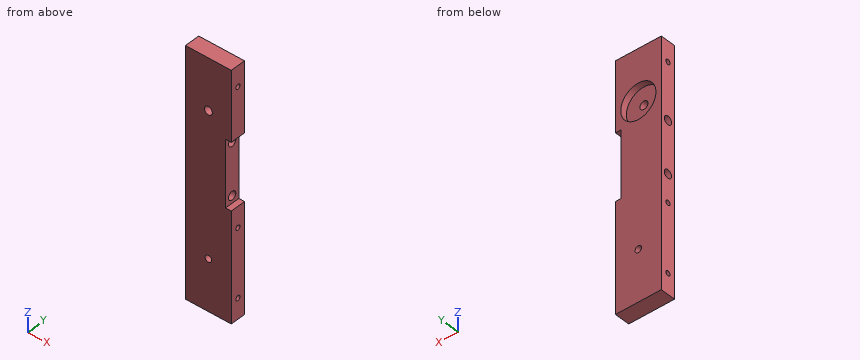
```python
from build123d import *

# Parameters (mm, degrees)
SKETCH2_W             = 28.575
SKETCH2_H             = 152.4
BOSS_EXTRUDE1_DEPTH   = 9.525
F_3_0MM_DOWEL_HOLE1_D = 3
LPATTERN1_COUNT       = 4
LPATTERN1_PITCH       = 42.333333333
SKETCH12_R            = 2.05
CUT_EXTRUDE1_DEPTH    = 156.348048749
SKETCH12_4_R          = 10.975
CUT_EXTRUDE2_DEPTH    = 4
SKETCH15_R            = 2.5
CUT_EXTRUDE3_DEPTH    = 156.154169296
SKETCH13_R            = 2.6
CUT_EXTRUDE4_DEPTH    = 156.348048749
SKETCH17_W            = 41.28
SKETCH17_H            = 9.525
CUT_EXTRUDE5_DEPTH    = 3.575


with BuildPart() as part:
    # Sketch2 → Boss-Extrude1 (new body)
    with BuildSketch(Plane(origin=(0, 0, 0), x_dir=(1, 0, 0), z_dir=(0, 1, 0))):
        with Locations((14.2875, 76.2)):
            Rectangle(SKETCH2_W, SKETCH2_H)
    extrude(amount=BOSS_EXTRUDE1_DEPTH)

    # Ø3.0mm Dowel Hole1 (through all)
    with Locations(Plane.ZY):
        with Locations((-139.7, 4.7625)):
            f_3_0mm_dowel_hole1 = Hole(F_3_0MM_DOWEL_HOLE1_D / 2)

    # LPattern1: Ø3.0mm Dowel Hole1 ×4, 1 skipped
    with Locations(*[(0, 0, i * LPATTERN1_PITCH) for i in range(1, LPATTERN1_COUNT) if i not in (2,)]):
        add(f_3_0mm_dowel_hole1, mode=Mode.SUBTRACT)

    # Sketch12 → Cut-Extrude1 (cut, through all)
    with BuildSketch(Plane(origin=(0, 9.525, 0), x_dir=(1, 0, 0), z_dir=(0, 1, 0))):
        with Locations(Location((14.2875, 120.65, 0), (0, 0, 270))):
            Circle(SKETCH12_R)
    extrude(amount=-CUT_EXTRUDE1_DEPTH, mode=Mode.SUBTRACT)

    # Sketch12<4> → Cut-Extrude2 (cut)
    with BuildSketch(Plane(origin=(0, 9.525, 0), x_dir=(1, 0, 0), z_dir=(0, 1, 0))):
        with Locations(Location((14.2875, 31.75, 0), (0, 0, 270))):
            Circle(SKETCH12_4_R)
    extrude(amount=-CUT_EXTRUDE2_DEPTH, mode=Mode.SUBTRACT)

    # Sketch15 → Cut-Extrude3 (cut, through all)
    with BuildSketch(Plane(origin=(0, 5.525, 0), x_dir=(1, 0, 0), z_dir=(0, 1, 0))):
        with Locations(Location((14.2875, 31.75, 0), (0, 0, 270))):
            Circle(SKETCH15_R)
    extrude(amount=-CUT_EXTRUDE3_DEPTH, mode=Mode.SUBTRACT)

    # Sketch13 → Cut-Extrude4 (cut, through all)
    with BuildSketch(Plane.ZY):
        with Locations((-80, 4.7625)):
            Circle(SKETCH13_R)
        with Locations((-47.79, 4.7625)):
            Circle(SKETCH13_R)
    extrude(amount=-CUT_EXTRUDE4_DEPTH, mode=Mode.SUBTRACT)

    # Sketch17 → Cut-Extrude5 (cut)
    with BuildSketch(Plane.ZY.offset(-28.575)):
        with Locations((-63.895, 4.7625)):
            Rectangle(SKETCH17_W, SKETCH17_H)
    extrude(amount=CUT_EXTRUDE5_DEPTH, mode=Mode.SUBTRACT)


solid = part.part
```
Could you check a few things on this model? Use its own coordinates, in mm. Coordinates: 2 decimals unless noted, no trailing zeros. Order: outer loops, then holes, each group sorted by start corner. A loop starts at its lowest first (then second) coordinate and runs counter-clockwise, first axis right, second up. Notation, with made-up numbers: M 47.25,59.25 L 56.25,59.25 A32 ccw 56.25,97.25 Z; hole C 59,81 d2. An arc over 180 degrees is marked long. Use one line per item in the form item = value. Start each with the question number.
1. For pin 1 (11 mm diameter, centred on x = 14, z = -37, fed in from +Y) (3 decimals); pin 2 (5 mm diameter, centred on y = 4, z = -71, fed in from +X), each with a flat end and sliding along its axis, tell me the tip position at first contact or that it passes through.
2. Please list where these lines run through material, in increasing order: line 1 (Z direction, x = 24.25, y = 4.5); line 2 (Y direction, x = 14.5, z = -47.79) (1 decimal); line 3 (Y direction, x = 19.25, z = -12.7) (1 decimal).
3. Suppose I cut it at B-B on x = 9.25. Write out the boundary of the cut face in (y, z) (1 decimal), then the cut area to 3 significant figures.
4. Suppose I cut it at C-C on z = -31.75. Write out the boundary of the cut face in (x, y) (1 decimal).
5. Suppose I cut it at D-D on x = 19.75. Write out the boundary of the cut face in (y, z) (1 decimal), then the cut area to 3 significant figures.
6. Suppose I cut it at A-A on z = -139.7. Write out the boundary of the cut face in (x, y) (1 decimal), then the cut area to 3 significant figures.
Geometry says:
q1.pin_1 = 5.525
q1.pin_2 = 25
q2.line_1 = -152.4 to -141.18, -138.22 to -98.84, -95.89 to -82.59, -77.41 to -50.38, -45.2 to -14.18, -11.22 to 0
q2.line_2 = 0 to 2.2, 7.4 to 9.5
q2.line_3 = 0 to 3.3, 6.3 to 9.5
q3.outline = M 0,-152.4 L 9.5,-152.4 L 9.5,-41.5 L 5.5,-41.5 L 5.5,-22 L 9.5,-22 L 9.5,0 L 0,0 Z; hole C 4.8,-80 d5.2; hole C 4.8,-47.8 d5.2; hole C 4.8,-139.7 d3; hole C 4.8,-97.4 d3; hole C 4.8,-12.7 d3
q3.area = 1,310 mm^2
q4.outline = M 0,0 L 11.8,0 L 11.8,5.5 L 3.3,5.5 L 3.3,9.5 L 0,9.5 Z; M 16.8,0 L 28.6,0 L 28.6,9.5 L 25.3,9.5 L 25.3,5.5 L 16.8,5.5 Z
q5.outline = M 0,-152.4 L 9.5,-152.4 L 9.5,-41.3 L 5.5,-41.3 L 5.5,-22.2 L 9.5,-22.2 L 9.5,0 L 0,0 Z; hole C 4.8,-80 d5.2; hole C 4.8,-47.8 d5.2; hole C 4.8,-139.7 d3; hole C 4.8,-97.4 d3; hole C 4.8,-12.7 d3
q5.area = 1,310 mm^2
q6.outline = M 0,0 L 28.6,0 L 28.6,3.3 L 0,3.3 Z; M 0,6.3 L 28.6,6.3 L 28.6,9.5 L 0,9.5 Z
q6.area = 186 mm^2
